Here's how the part is built. I have some questions about the finished solid (model axes, mm). A direction names the side the tool comes from. Round coordinates to 2 decimals unless told otherwise and drop trailing zeros. Write each loop counter-clockwise with the first axis right and the second up, starting at its lowest first coordinate (ties: lowest second). Pieces come first, ordered by that corner, then holes. Notation, with made-up numbers: M 43,-30.75 L 79,-30.75 A16 cw 79,-8.75 Z; hole C 87.5,76.5 d3. An arc over 180 degrees is marked long. Use one line per item in the form item = value. Start each with the question number.
Q1. For faces 1 (the face through (-2.9, 0, 1.3)), 2 (the face through (-3.412, 3, 0)), which set-ups out of +Z, -Z, +X, -X, +Y, -Y let a thin tool reach every point of the face, with its end or its side?
Q2. I need wall thicknesses on line 1 along X through (y, z) = (3.5, 0); line 2 along Z through (x, y) = (-2.75, 4); line 3 along Z through (x, y) = (-0.5, 1). Which ranges of each line are inside material? Lowest first, please. Write a range as from..to.
Q3. We'd pull the mould along Z, two halves only. Please class faces 3 (the face through (-1.38, 3.13, 6.2)), 4 (the face through (-2.9, 6.35, 1.3)), 5 (the face through (-3, 3, 1)): +Z half, -Z half, draft (parallel to the pull), parting line (faces both ways), or undercut.
Q4. I'm going to push flat-ended pins straight in: pin 1 Ø1.2 at (x, y) = (-3, 2) entering from -Z; pin 2 Ø1.5 at (y, z) = (2.5, 3) entering from +X; pin 3 Ø1.2 at (x, y) = (-3, 4) entering from +Z. Where does each tip first touch, or does it pass through?
Q5. I want a section at B-B on z = 0. List the corners of the cut face in (x, y) for me, and give its area (3 significant figures).
Q6. I want a section at A-A on y = 5.75. List the corners of the cut face in (x, z) for me, and give its area (3 significant figures).
Q7. I want a section at D-D on z = 5. List the corners of the cut face in (x, y) for me, and give its area (3 significant figures).
Q8. I want a section at C-C on x = 0. List the corners of the cut face in (y, z) for me.
```python
from build123d import *

# Parameters (mm, degrees)
SKETCH1_R           = 6.35
BOSS_EXTRUDE1_DEPTH = 6.35
SKETCH2_R           = 4
CUT_EXTRUDE1_DEPTH  = 6.35
SKETCH3_W           = 2
SKETCH3_H           = 2
CUT_EXTRUDE2_DEPTH  = 6.35


with BuildPart() as part:
    # Sketch1 → Boss-Extrude1 (new body)
    with BuildSketch(Plane(origin=(0, 0, 0), x_dir=(1, 0, 0), z_dir=(0, 1, 0))):
        Circle(SKETCH1_R)
    extrude(amount=BOSS_EXTRUDE1_DEPTH)

    # Sketch2 → Cut-Extrude1 (cut)
    with BuildSketch(Plane(origin=(0, 6.35, 0), x_dir=(1, 0, 0), z_dir=(0, 1, 0))):
        with Locations((1.5875, 0)):
            Circle(SKETCH2_R)
    extrude(amount=-CUT_EXTRUDE1_DEPTH, mode=Mode.SUBTRACT)

    # Sketch3 → Cut-Extrude2 (cut)
    with BuildSketch(Plane(origin=(0, 6.35, 0), x_dir=(1, 0, 0), z_dir=(0, 1, 0))):
        with Locations((-2.4125, 0)):
            Rectangle(SKETCH3_W, SKETCH3_H)
    extrude(amount=-CUT_EXTRUDE2_DEPTH, mode=Mode.SUBTRACT)


solid = part.part
```
Reported:
q1.face_1 = +Z, -Z, +X, -X, -Y
q1.face_2 = +Y, -Y
q2.line_1 = -6.35..-3.41, 5.59..6.35
q2.line_2 = -5.72..-1, 1..5.72
q2.line_3 = -6.33..-3.41, 3.41..6.33
q3.face_3 = parting line
q3.face_4 = draft
q3.face_5 = undercut
q4.pin_1 = -5.88
q4.pin_2 = 5.94
q4.pin_3 = 5.88
q5.outline = M -6.35,0 L -3.41,0 L -3.41,6.35 L -6.35,6.35 Z; M 5.59,0 L 6.35,0 L 6.35,6.35 L 5.59,6.35 Z
q5.area = 23.5 mm^2
q6.outline = C 0,0 d12.7; hole M -3.41,-1 L -2.29,-1 A4 ccw long -2.29,1 L -3.41,1 Z
q6.area = 74.3 mm^2
q7.outline = M -3.91,0 L 3.91,0 L 3.91,6.35 L -3.91,6.35 Z
q7.area = 49.7 mm^2
q8.outline = M 0,-6.35 L 6.35,-6.35 L 6.35,-3.67 L 0,-3.67 Z; M 0,3.67 L 6.35,3.67 L 6.35,6.35 L 0,6.35 Z
